```python
from build123d import *

# Parameters (mm, degrees)
PAD_DEPTH    = 10
SKETCH001_R  = 12.386876
SKETCH001_W  = 52.232122
SKETCH001_H  = 12.547379
PAD001_DEPTH = 10


with BuildPart() as part:
    # Sketch → Pad (new body)
    with BuildSketch(Plane.XY):
        Polygon((30.372211, -55.345623), (63.116821, -1.369705), (32.74461, 53.975918), (-30.372211, 55.345623), (-63.116821, 1.369705), (-32.74461, -53.975918), align=None)
    extrude(amount=PAD_DEPTH)

    # Sketch001 (on Face8 of Pad) → Pad001 (join)
    with BuildSketch(Plane.XY.offset(10)):
        with Locations((30.440666, -7.472315)):
            Circle(SKETCH001_R)
        with Locations((1.698405, 30.315723)):
            Rectangle(SKETCH001_W, SKETCH001_H)
        Polygon((-17.414461, -33.150673), (-10.291936, -23.310478), (-15.252532, -12.222093), (-27.335653, -10.973903), (-34.458178, -20.814098), (-29.497582, -31.902483), align=None)
    extrude(amount=PAD001_DEPTH)


solid = part.part
```
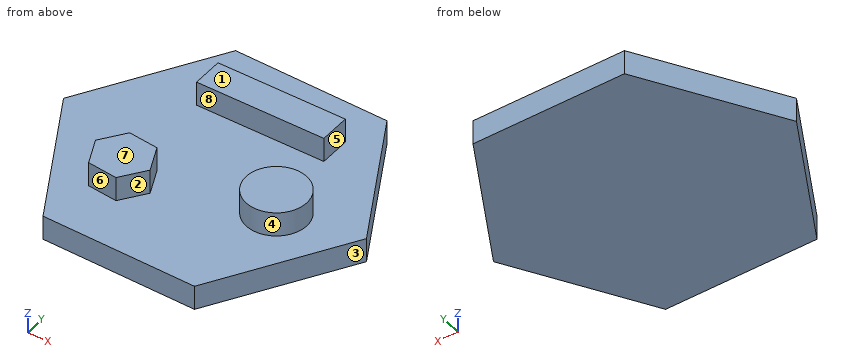
Here's how the part is built. I have some questions about the finished solid (model axes, mm). Face numbers are marked on the shaded views. A direction names the side the tool comes from. Coordinates: 2 decimals unless noted, no trailing zeros. Write each loop counter-clockwise with the first axis right and the second up, starting at its lowest first coordinate (ties: lowest second). Pieces come first, ordered by that corner, then holes. Notation, with made-up numbers: (80, 22) -> (134, 22) arc R24 ccw to (134, 51) -> close; hole circle Ø7 at (8.5, -18). An arc over 180 degrees is marked (long way). Use a Markdown table: item, result. Add a question column.
(1) Please list where these lines run through material, in increasing order: line 1 (X direction, y = 27.5, z = 17); line 2 (Z direction, x = -11, y = -49.5); line 3 (Y direction, x = 7.5, z = 16.75).
(2) If we section it at B-B, the plane z = 6.5: Write out the boundary of the cut face in (x, y), and give its area (3 significant figures).
(3) For the marked faces 1, 2, 3, 4 and 5, which set-ups out of +Z, -Z, +X, -X, +Y, -Y let a thin tool reach every point of the face, with its end or its side?
(4) If we section it at D-D, the plane x = 21.5: Write out the boundary of the cut face in (y, z), and give its area (3 significant figures).
(5) We'd pull the mould along Y, two halves only. Please class the marked faces 6, 7 and 8: +Y half, -Y half, draft (parallel to the pull), parting line (faces both ways), or undercut.
(6) If we section it at A-A, the plane z = 14.5: Write out the boundary of the cut face in (x, y).
(7) I'm going to push flat-ended pins straight in: P1, Ø8, axis at x = 14.5, z = 15, coming from the +Y side; P2, Ø1.5, axis at y = -9.5, z = 2.5, coming from the +X side; P3, Ø2, axis at y = 31, z = 9, coming from the -X side. Where does each tip first touch, or does it pass through?
(8) If we section it at C-C, the plane y = -15: Write out the boundary of the cut face in (x, z), and give its area (3 significant figures).
Outcome:
| question | item | result |
|---|---|---|
| 1 | line 1 | x = -24.42 to 27.81 |
| 1 | line 2 | z = 0 to 10 |
| 1 | line 3 | y = 24.04 to 36.59 |
| 2 | outline | (-63.12, 1.37) -> (-32.74, -53.98) -> (30.37, -55.35) -> (63.12, -1.37) -> (32.74, 53.98) -> (-30.37, 55.35) -> close |
| 2 | area | 10,400 mm^2 |
| 3 | face 1 | +Z, +X, -X, +Y, -Y |
| 3 | face 2 | +Z, +X, -Y |
| 3 | face 3 | +Z, -Z, +X, -Y |
| 3 | face 4 | +Z |
| 3 | face 5 | +Z, +X, +Y |
| 4 | outline | (-55.15, 0) -> (54.22, 0) -> (54.22, 10) -> (36.59, 10) -> (36.59, 20) -> (24.04, 20) -> (24.04, 10) -> (1.1, 10) -> (1.1, 20) -> (-16.05, 20) -> (-16.05, 10) -> (-55.15, 10) -> close |
| 4 | area | 1,390 mm^2 |
| 5 | face 6 | -Y half |
| 5 | face 7 | draft |
| 5 | face 8 | undercut |
| 6 | outline | (-34.46, -20.81) -> (-29.5, -31.9) -> (-17.41, -33.15) -> (-10.29, -23.31) -> (-15.25, -12.22) -> (-27.34, -10.97) -> close; (-24.42, 24.04) -> (27.81, 24.04) -> (27.81, 36.59) -> (-24.42, 36.59) -> close; circle Ø24.77 at (30.44, -7.47) |
| 7 | P1 | stops at y = 36.59 |
| 7 | P2 | stops at x = 58.64 |
| 7 | P3 | stops at x = -45.75 |
| 8 | outline | (-54.13, 0) -> (54.85, 0) -> (54.85, 10) -> (40.28, 10) -> (40.28, 20) -> (20.6, 20) -> (20.6, 10) -> (-14.01, 10) -> (-14.01, 20) -> (-30.25, 20) -> (-30.25, 10) -> (-54.13, 10) -> close |
| 8 | area | 1,450 mm^2 |
